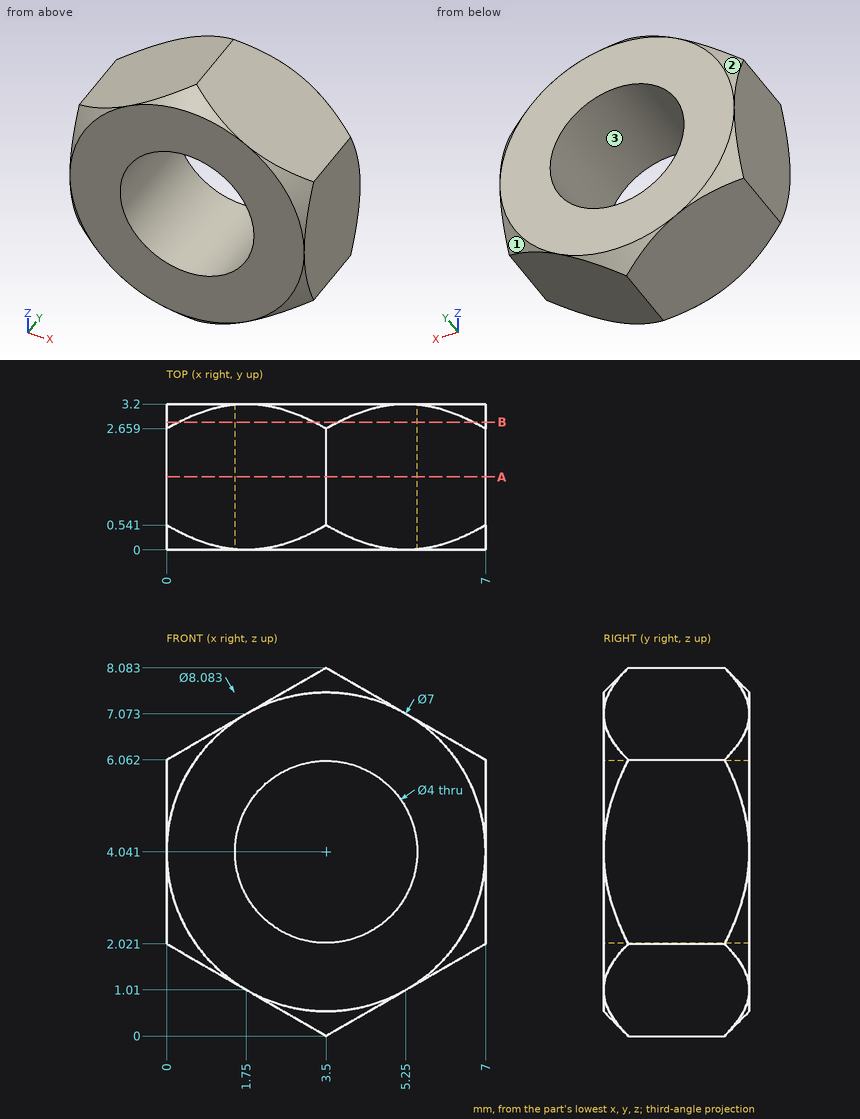
The drawing under review shows one solid part. Ordinate dimensions are in mm from its lowest x, y, z. Coordinates: 2 decimals unless noted, no trailing zeros. Order: outer loops, then holes, each group sorted by start corner. A loop starts at its lowest first (then second) coordinate and runs counter-clockwise, first axis right, second up. Notation, with made-up numbers: (-8.75, 14) -> (38.25, 14) arc R38 ccw to (38.25, 53) -> close; hole circle Ø6 at (-19, 59). An arc over 180 degrees is marked (long way). Answer in a Markdown table with one row per item.
(1) Consider section A-A (y = 1.6). Write out the cut boundary in (x, z).
Answers:
| item | result |
|---|---|
| outline | (0, 2.02) -> (3.5, 0) -> (7, 2.02) -> (7, 6.06) -> (3.5, 8.08) -> (0, 6.06) -> close; hole circle Ø4 at (3.5, 4.04) |
(2) Wall thickness on line 1 along X through (y, z) = (0.4, 3.75); line 2 along Z through (x, y) = (3, 2.4) (1 decimal); line 3 along Z through (x, y) = (2.25, 2) (1 decimal): over which ranges is each line inside the solid? List them lowest first.
Answers:
| item | result |
|---|---|
| line 1 | 0 to 1.52, 5.48 to 7 |
| line 2 | 0.3 to 2.1, 6 to 7.8 |
| line 3 | 0.7 to 2.5, 5.6 to 7.4 |
(3) The part is to be moulded in two halves that separate along X. For the marked faces 1, 2 and 3, say which applies: +X half, -X half, draft (parallel to the pull), parting line (faces both ways), or undercut.
Answers:
| item | result |
|---|---|
| face 1 | +X half |
| face 2 | -X half |
| face 3 | undercut |
(4) Consider section B-B (y = 2.8). Write out the cut boundary in (x, z).
Answers:
| item | result |
|---|---|
| outline | (0, 2.32) arc R3.9 ccw to (0.26, 1.87) -> (3.24, 0.15) arc R3.9 ccw to (3.76, 0.15) -> (6.74, 1.87) arc R3.9 ccw to (7, 2.32) -> (7, 5.76) arc R3.9 ccw to (6.74, 6.21) -> (3.76, 7.93) arc R3.9 ccw to (3.24, 7.93) -> (0.26, 6.21) arc R3.9 ccw to (0, 5.76) -> close; hole circle Ø4 at (3.5, 4.04) |
